The listing builds one solid part. Answer for the finished solid, in the listing's coordinates (mm). Face numbers are marked on the shaded views. A direction names the side the tool comes from. Give positions to 0.01 mm unless a question says otherwise; leave off trailing zeros. Loops run counter-clockwise (first coordinate to the right, second up) from the corner with the lowest first, then second, coordinate; pieces in that order, holes last.
Item 1: The mould has two halves that part along X. Classify the marked faces 1, 2 and 3: pulls with the +X half, pulls with the -X half, needs draft (parallel to the pull), parting line crosses it, or undercut.
Item 2: Section D-D, the plane z = 21.5 is taken. Give the vertices of the cut face in (x, y), and give its area (3 significant figures).
Item 3: A tool of negligible diameter and unlimited length cuts with its end or side. For the marked faces 4, 5, 6, 7 and 8, from which of +Z, -Z, +X, -X, +Y, -Y can it reach the whole face along a straight path? Write none if from no direction.
Item 4: Section B-B, the plane y = -115 is taken. Give the vertices of the cut face in (x, z).
Item 5: Section A-A, the plane z = 0 is taken. Give the number of separate pieces and of enclosed holes in the cut face, and give its area (3 significant figures).
Item 6: Each of these flat-tipped pins is pushed along its axis until it touches: pin 1 Ø7.5 at (y, z) = (-85, 1.5) entering from +X; pin 2 Ø12.5 at (y, z) = (28.575, 0) entering from +X; pin 3 Ø12 at (x, z) = (2, -36.5) entering from +Y; pin 4 Ø1 at (x, y) = (-6.5, -125) entering from +Z. Where does it stop, or does it pass through?
Item 7: Consider line 1 along Z through (x, y) = (12, -112); line 2 along X through (y, z) = (12, -11); line 3 along Y through (x, z) = (-16.5, 16). Determine where each line is inside the solid, lowest interval first.
Item 8: Section C-C, the plane x = 10 is taken. Give the vertices of the cut face in (y, z).
from build123d import *

# Parameters (mm, degrees)
F1_DEPTH  = 203.2
F3_DEPTH  = 38.1
F5_DEPTH  = 50.8
F6_DEPTH  = 50.8
F7_R      = 4.7625
F8_DEPTH  = 63.5
F9_R      = 6.35
F10_R     = 6.35
F11_DEPTH = 25.4


with BuildPart() as f1:
    # F0 (on Front) → F1 (new body)
    with BuildSketch(Plane.XZ):
        with BuildLine():
            Line((-12.7, -19.05), (12.7, -19.05))
            ThreePointArc((12.7, -19.05), (17.1901280605, -17.1901280605), (19.05, -12.7))
            Line((19.05, -12.7), (19.05, 12.7))
            ThreePointArc((19.05, 12.7), (17.1901280605, 17.1901280605), (12.7, 19.05))
            Line((12.7, 19.05), (-12.7, 19.05))
            ThreePointArc((-12.7, 19.05), (-17.1901280605, 17.1901280605), (-19.05, 12.7))
            Line((-19.05, 12.7), (-19.05, -12.7))
            ThreePointArc((-19.05, -12.7), (-17.1901280605, -17.1901280605), (-12.7, -19.05))
        make_face()
    extrude(amount=F1_DEPTH)

    # F2 (on face) → F3 (cut)
    with BuildSketch(Plane.YZ.offset(19.05)):
        with BuildLine():
            Line((-177.8, -6.35), (-101.6, -6.35))
            ThreePointArc((-101.6, -6.35), (-95.25, 0), (-101.6, 6.35))
            Line((-101.6, 6.35), (-177.8, 6.35))
            ThreePointArc((-177.8, 6.35), (-184.15, 0), (-177.8, -6.35))
        make_face()
    extrude(amount=-F3_DEPTH, mode=Mode.SUBTRACT)

    # F4 (on Top) → F5 (join)
    with BuildSketch(Plane.XY):
        with BuildLine():
            ThreePointArc((-31.75, 6.35), (-29.8901280605, 1.8598719395), (-25.4, 0))
            Line((-25.4, 0), (25.4, 0))
            ThreePointArc((25.4, 0), (29.8901280605, 1.8598719395), (31.75, 6.35))
            Line((31.75, 6.35), (31.75, 50.8))
            Line((31.75, 50.8), (25.4, 50.8))
            Line((25.4, 50.8), (25.4, 12.7))
            ThreePointArc((25.4, 12.7), (23.5401280605, 8.2098719395), (19.05, 6.35))
            Line((19.05, 6.35), (-19.05, 6.35))
            ThreePointArc((-19.05, 6.35), (-23.5401280605, 8.2098719395), (-25.4, 12.7))
            Line((-25.4, 12.7), (-25.4, 50.8))
            Line((-25.4, 50.8), (-31.75, 50.8))
            Line((-31.75, 50.8), (-31.75, 6.35))
        make_face()
    extrude(amount=F5_DEPTH)

    # F6 (add): a face of the model
    f6_faces = [f1.faces().sort_by_distance(p)[0] for p in [
        (-26.2131967782, 31.75, 0),
    ]]
    extrude(f6_faces, amount=F6_DEPTH)

    # F7 (on face) → F8 (cut)
    with BuildSketch(Plane.YZ.offset(31.75)):
        with Locations((28.575, 38.1)):
            Circle(F7_R)
        with Locations((28.575, 19.05)):
            Circle(F7_R)
        with Locations((28.575, 0)):
            Circle(F7_R)
        with Locations((28.575, -19.05)):
            Circle(F7_R)
        with Locations((28.575, -38.1)):
            Circle(F7_R)
    extrude(amount=-F8_DEPTH, mode=Mode.SUBTRACT)

    # F9
    f9_edges = [f1.edges().sort_by_distance(p)[0] for p in [
        (28.575, 50.8, 50.8),
        (-28.575, 50.8, 50.8),
        (-28.575, 50.8, -50.8),
        (28.575, 50.8, -50.8),
    ]]
    fillet(f9_edges, radius=F9_R)

    # F10 (on face) → F11 (cut)
    with BuildSketch(Plane(origin=(0, 0, -19.05), x_dir=(1, 0, 0), z_dir=(0, 0, -1))):
        with Locations((0, 19.05)):
            Circle(F10_R)
    extrude(amount=-F11_DEPTH, mode=Mode.SUBTRACT)


solid = f1.part
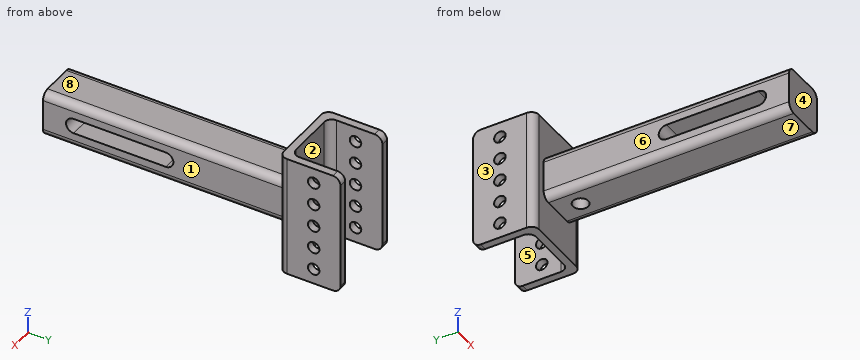
Worked answers:
1. face 1: pulls with the +X half
1. face 2: undercut
1. face 3: pulls with the -X half
2. outline: (-31.75, 6.35) arc R6.35 ccw to (-25.4, 0) - (25.4, 0) arc R6.35 ccw to (31.75, 6.35) - (31.75, 24.49) - (25.4, 24.49) - (25.4, 12.7) arc R6.35 cw to (19.05, 6.35) - (-19.05, 6.35) arc R6.35 cw to (-25.4, 12.7) - (-25.4, 24.49) - (-31.75, 24.49) - close; (-31.75, 32.66) - (-25.4, 32.66) - (-25.4, 50.8) - (-31.75, 50.8) - close; (25.4, 32.66) - (31.75, 32.66) - (31.75, 50.8) - (25.4, 50.8) - close
2. area: 864 mm2
3. face 4: +Z, -Z, +X, -X, -Y
3. face 5: +Z, -Z, +Y
3. face 6: +Z, -Z, -X, -Y
3. face 7: -Z, +X, -X, -Y
3. face 8: +Z, +X, -X, -Y
4. outline: (-19.05, -12.7) arc R6.35 ccw to (-12.7, -19.05) - (12.7, -19.05) arc R6.35 ccw to (19.05, -12.7) - (19.05, -6.35) - (-19.05, -6.35) - close; (-19.05, 6.35) - (19.05, 6.35) - (19.05, 12.7) arc R6.35 ccw to (12.7, 19.05) - (-12.7, 19.05) arc R6.35 ccw to (-19.05, 12.7) - close
5. separate pieces: 4
5. enclosed holes: 1
5. area: 5,070 mm2
6. pin 1: stops at x = 19.05
6. pin 2: stops at x = 31.75
6. pin 3: stops at y = 6.35
6. pin 4: stops at z = 19.05
7. line 1: z = -19.05 to -6.35, 6.35 to 19.05
7. line 2: x = -31.75 to -25.36, 25.36 to 31.75
7. line 3: y = -203.2 to 6.35
8. outline: (-203.2, -19.05) - (0, -19.05) - (0, -50.8) - (6.35, -50.8) - (6.35, 50.8) - (0, 50.8) - (0, 19.05) - (-203.2, 19.05) - close; hole (-177.8, -6.35) - (-101.6, -6.35) arc R6.35 ccw to (-101.6, 6.35) - (-177.8, 6.35) arc R6.35 ccw to start
